from build123d import *

# Parameters (mm, degrees)
EXTRUDE_1_DEPTH     = 3
SKETCH_1_3_W        = 9.5
SKETCH_1_3_H        = 3.25
EXTRUDE_2_DEPTH     = 3
SKETCH_1_4_R        = 1.5
CUT_EXTRUDE_1_DEPTH = 3
CUT_EXTRUDE_2_DEPTH = 3
SKETCH_3_W          = 11.590372196
SKETCH_3_H          = 9.306034482
EXTRUDE_3_DEPTH     = 13
SKETCH_4_R          = 2.5
EXTRUDE_4_DEPTH     = 15
FILLET_1_R          = 3


with BuildPart() as part:
    # Sketch 1 → Extrude 1 (new body)
    with BuildSketch(Plane(origin=(0, 0, 0), x_dir=(1, 0, 0), z_dir=(0, 1, 0))):
        with BuildLine():
            Line((-9.33144513, 4.653017241), (7.66855487, 4.653017241))
            ThreePointArc((7.66855487, 4.653017241), (12.321572111, 0), (7.66855487, -4.653017241))
            Line((7.66855487, -4.653017241), (-9.33144513, -4.653017241))
            ThreePointArc((-9.33144513, -4.653017241), (-13.984462372, 0), (-9.33144513, 4.653017241))
        make_face()
    extrude(amount=EXTRUDE_1_DEPTH)

    # Sketch 1_3 → Extrude 2 (add)
    with BuildSketch(Plane(origin=(0, 0, 0), x_dir=(1, 0, 0), z_dir=(0, 1, 0))):
        with Locations((-0.83144513, 1.625)):
            Rectangle(SKETCH_1_3_W, SKETCH_1_3_H)
        with Locations((-0.83144513, -1.625)):
            Rectangle(SKETCH_1_3_W, SKETCH_1_3_H)
    extrude(amount=-EXTRUDE_2_DEPTH)

    # Sketch 1_4 → Cut-Extrude 1 (cut)
    with BuildSketch(Plane(origin=(0, 0, 0), x_dir=(1, 0, 0), z_dir=(0, 1, 0))):
        with Locations(Location((-9.33144513, 0, 0), (0, 0, 270))):
            Circle(SKETCH_1_4_R)
        with Locations(Location((7.66855487, 0, 0), (0, 0, 270))):
            Circle(SKETCH_1_4_R)
    extrude(amount=CUT_EXTRUDE_1_DEPTH, mode=Mode.SUBTRACT)

    # Sketch 2 → Cut-Extrude 2 (cut)
    with BuildSketch(Plane.XZ.offset(3)):
        Polygon((-4.58144513, 1.75), (2.91855487, 1.75), (2.301410437, -1.75), (-3.964300698, -1.75), align=None)
    extrude(amount=-CUT_EXTRUDE_2_DEPTH, mode=Mode.SUBTRACT)

    # Sketch 3 → Extrude 3 (add)
    with BuildSketch(Plane(origin=(0, 3, 0), x_dir=(1, 0, 0), z_dir=(0, 1, 0))):
        with Locations((-0.00308465, 0)):
            Rectangle(SKETCH_3_W, SKETCH_3_H)
    extrude(amount=EXTRUDE_3_DEPTH)

    # Sketch 4 → Extrude 4 (add)
    with BuildSketch(Plane(origin=(0, 16, 0), x_dir=(1, 0, 0), z_dir=(0, 1, 0))):
        with Locations(Location((0, 0, 0), (0, 0, 270))):
            Circle(SKETCH_4_R)
    extrude(amount=EXTRUDE_4_DEPTH)

    # Fillet 1
    fillet_1_edges = [part.edges().sort_by_distance(p)[0] for p in [
        (0, 16, -2.5),
    ]]
    fillet(fillet_1_edges, radius=FILLET_1_R)


solid = part.part
Geometry check sheet. Reference: the model listing, model coordinates, mm. A direction names the side the tool comes from. Give positions to 0.01 mm unless a question says otherwise; leave off trailing zeros. Write each loop counter-clockwise with the first axis right and the second up, starting at its lowest first coordinate (ties: lowest second). Pieces come first, ordered by that corner, then holes. Notation, with made-up numbers: M 68.5,45 L 110.5,45 A17 ccw 110.5,60 Z; hole C -18.5,73 d6. An arc over 180 degrees is marked long. One line per question, with ' | ' between items.
1. Scan lines: line 1 along X through (y, z) = (1.65, 0); line 2 along Z through (x, y) = (-9.5, 2); line 3 along Y through (x, z) = (11, -0.25). Record each from-to range of solid material in increasing order. Write a range as from..to.
Ans:
line 1: -13.98..-10.83, -7.83..6.17, 9.17..12.32 | line 2: -4.65..-1.49, 1.49..4.65 | line 3: 0..3
2. Cross-section at A-A (z = 0). Count the separate pieces of the cut face and the enclosed holes in it, plus the area to 3 significant figures.
Ans:
separate pieces: 3 | enclosed holes: 0 | area: 298 mm2
3. Mould release check, pull along Z, two halves, no side actions. Record for faces 1 (the face through (-8.07, 1.48, 0.81)), 2 (the face through (12.32, 1.48, -0.1)), 3 (the face through (-5.798, 9, 0)): released by +Z, released by -Z, zero draft, split by the parting line, or undercut.
Ans:
face 1: undercut | face 2: split by the parting line | face 3: zero draft
4. Gauge pin test, flat ends, axial feed: pin 1 (4.5 mm diameter, centred on y = 11.5, z = 0.5, fed in from -X); pin 2 (1 mm diameter, centred on y = 26.5, z = 1, fed in from +X); pin 3 (1.5 mm diameter, centred on y = 21.5, z = -0.5, fed in from +X). Record the tip position at first contact, or that the pin passes through.
Ans:
pin 1: x = -5.8 | pin 2: x = 2.45 | pin 3: x = 2.5
5. Set-up check for faces 4 (the face through (-5.581, -1, 0)), 5 (the face through (-5.646, 16, 0.323)), 6 (the face through (2.614, -1.521, 0.024)), 7 (the face through (0.751, 24.832, 2.385)): record each of +Z, -Z, +X, -X, +Y, -Y from which the full face is reachable in a straight line by a thin tool's end or side.
Ans:
face 4: +Z, -Z, -X, -Y | face 5: -X, +Y | face 6: -Y | face 7: +Y
6. Cross-section at B-B (y = 10). Enter the section's corners in (x, z), plus the area to 3 significant figures.
Ans:
outline: M -5.8,-4.65 L 5.79,-4.65 L 5.79,4.65 L -5.8,4.65 Z | area: 108 mm2
7. Cross-section at C-C (y = 25.5). Enter the section's corners in (x, z), plus the area to 3 significant figures.
Ans:
outline: C 0,0 d5 | area: 19.6 mm2
